```python
from build123d import *

# Parameters (mm, degrees)
BOSS_EXTRUDE1_DEPTH = 6
SKETCH2_W           = 8
SKETCH2_H           = 3
CUT_EXTRUDE1_DEPTH  = 17.027339923
SKETCH3_W           = 3.2
SKETCH3_H           = 3.2
CUT_EXTRUDE2_DEPTH  = 5
FILLET1_R           = 2.5
FILLET2_R           = 5
FILLET3_R           = 1
CHAMFER1_SIZE       = 0.5
CHAMFER2_SIZE       = 1


with BuildPart() as part:
    # Sketch1 → Boss-Extrude1 (new body)
    with BuildSketch(Plane.XY):
        with BuildLine():
            Line((5.475, -93.5), (-8.525, -93.5))
            ThreePointArc((-8.525, -93.5), (-12.525, -89.5), (-8.525, -85.5))
            Line((-8.525, -85.5), (5.475, -85.5))
            ThreePointArc((5.475, -85.5), (9.475, -89.5), (5.475, -93.5))
        make_face()
    extrude(amount=BOSS_EXTRUDE1_DEPTH)

    # Sketch2 → Cut-Extrude1 (cut, through all)
    with BuildSketch(Plane.XZ.offset(93.5)):
        with Locations((-8.525, 4.5)):
            Rectangle(SKETCH2_W, SKETCH2_H)
        with Locations((5.475, 4.5)):
            Rectangle(SKETCH2_W, SKETCH2_H)
    extrude(amount=-CUT_EXTRUDE1_DEPTH, mode=Mode.SUBTRACT)

    # Sketch3 → Cut-Extrude2 (cut)
    with BuildSketch(Plane(origin=(0, 0, 0), x_dir=(-1, 0, 0), z_dir=(0, 0, -1))):
        with Locations((1.525, -89.5)):
            Rectangle(SKETCH3_W, SKETCH3_H)
    extrude(amount=-CUT_EXTRUDE2_DEPTH, mode=Mode.SUBTRACT)

    # Fillet1
    fillet1_edges = [part.edges().sort_by_distance(p)[0] for p in [
        (-4.525, -89.5, 6),
        (1.475, -89.5, 6),
    ]]
    fillet(fillet1_edges, radius=FILLET1_R)

    # Fillet2
    fillet2_edges = [part.edges().sort_by_distance(p)[0] for p in [
        (1.475, -89.5, 3),
        (-4.525, -89.5, 3),
    ]]
    fillet(fillet2_edges, radius=FILLET2_R)

    # Fillet3
    fillet3_edges = [part.edges().sort_by_distance(p)[0] for p in [
        (-5.788932023, -93.5, 3.527864045),
        (-5.788932023, -85.5, 3.527864045),
        (-12.525, -89.5, 3),
        (-8.275, -85.5, 3),
        (-8.275, -93.5, 3),
        (9.475, -89.5, 3),
        (-1.525, -93.5, 6),
        (-3.143033989, -93.5, 5.736067977),
        (-1.525, -85.5, 6),
        (0.093033989, -85.5, 5.736067977),
        (5.225, -85.5, 3),
        (5.225, -93.5, 3),
        (0.093033989, -93.5, 5.736067977),
        (-3.143033989, -85.5, 5.736067977),
        (2.738932023, -93.5, 3.527864045),
        (2.738932023, -85.5, 3.527864045),
    ]]
    fillet(fillet3_edges, radius=FILLET3_R)

    # Chamfer1
    chamfer1_edges = [part.edges().sort_by_distance(p)[0] for p in [
        (-1.525, -93.5, 0),
        (-12.525, -89.5, 0),
        (-1.525, -85.5, 0),
        (9.475, -89.5, 0),
    ]]
    chamfer(chamfer1_edges, length=CHAMFER1_SIZE)

    # Chamfer2
    chamfer2_edges = [part.edges().sort_by_distance(p)[0] for p in [
        (0.075, -89.5, 5),
        (-1.525, -87.9, 5),
        (-3.125, -89.5, 5),
        (-1.525, -91.1, 5),
    ]]
    chamfer(chamfer2_edges, length=CHAMFER2_SIZE)


solid = part.part
```
Input: part model. Units: mm. Frame: model coordinates. A direction names the side the tool comes from. Give positions to 0.01 mm unless a question says otherwise; leave off trailing zeros. Order: outer loops, then holes, each group sorted by start corner. A loop starts at its lowest first (then second) coordinate and runs counter-clockwise, first axis right, second up. Notation, with made-up numbers: M 67,61.5 L 83,61.5 A19 ccw 83,68.5 Z; hole C 89.25,34 d9. An arc over 180 degrees is marked long. One line per question, with ' | ' between items. Start each with the question number.
1. Pull-direction query (Y, two-part tool) for faces 1 (the face through (9.474, -89.412, 1.24)), 2 (the face through (-0.321, -89.522, 4.396)), 3 (the face through (-9, -90, 3)), 4 (the face through (-2.729, -89.522, 4.396)); classes: released by +Y, released by -Y, zero draft, split by the parting line, or undercut.
2. Material intervals for probe 1 along Z at (x, y) = (5.75, -89.5); probe 2 along X at (y, z) = (-90.25, 0.75) (3 decimals); probe 3 along X at (y, z) = (-88.5, 4.5) (3 decimals), sorted ascending. Write a range as [from, to].
3. Access query for faces 5 (the face through (-1.5, -90.7, 4.4)), 6 (the face through (5.228, -85.785, 2.699)), 7 (the face through (5.222, -93.215, 2.699)). Directions: +Z, -Z, +X, -X, +Y, -Y. A direction counts if a zero-diameter tool reaches every point of the face in a straight line with its end or side. Return the directions, or none.
4. Section query A-A (x = -1.25). Return the cut outline in (y, z), and give its area (3 significant figures).
5. First-contact query: pin 1 Ø1.5 at (y, z) = (-92.5, 2) entering from -X; pin 2 Ø3 at (x, y) = (7, -89) entering from +Z; pin 3 Ø1.5 at (y, z) = (-91, 5.5) entering from -X. Flat tips, straight axial feed; report the tip coordinate or a pass-through.
Here are the results:
1) face 1: split by the parting line | face 2: undercut | face 3: zero draft | face 4: undercut
2) probe 1: [0, 3] | probe 2: [-12.454, -3.125], [0.075, 9.404] | probe 3: [-4.454, -2.625], [-0.425, 1.404]
3) face 5: -Z | face 6: +Z, +X, +Y | face 7: +Z, +X, -Y
4) outline: M -93.5,0.5 L -93,0 L -91.1,0 L -91.1,4 L -90.1,5 L -88.9,5 L -87.9,4 L -87.9,0 L -86,0 L -85.5,0.5 L -85.5,5 A1 ccw -86.5,6 L -92.5,6 A1 ccw -93.5,5 Z | area: 32.3 mm²
5) pin 1: x = -11.83 | pin 2: z = 3 | pin 3: x = -4.23
